Can you work these out from the model? Positions are in its coordinate system, mm. Face numbers are marked on the shaded views. A direction names the side the tool comes from. Round coordinates to 2 decimals unless told otherwise and drop trailing zeros. Order: outer loops, then holes, each group sorted by start corner. A loop starts at its lowest first (then second) coordinate and runs counter-clockwise, first axis right, second up. Notation, with made-up numbers: (-18.75, 69) - (35.25, 69) arc R15 cw to (35.25, 77) - close; hole circle Ø9 at (40, 73.25). An arc over 180 degrees is marked (long way). Write item = value, one per line.
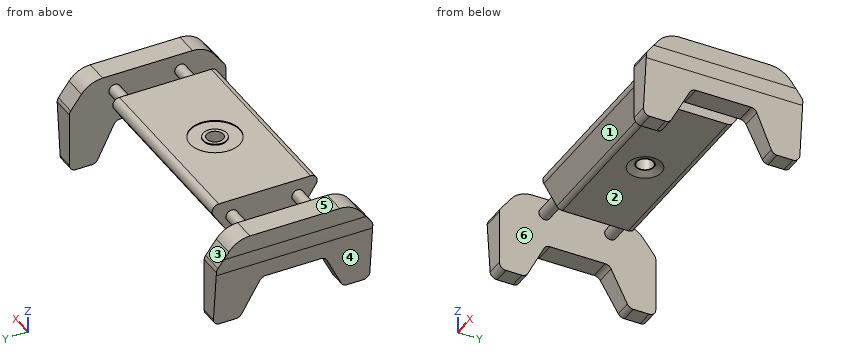
from build123d import *

# Parameters (mm, degrees)
BOSS_EXTRUDE1_DEPTH     = 56
SKETCH2_R               = 1.75
BOSS_EXTRUDE2_DEPTH     = 10
BOSS_EXTRUDE3_DEPTH     = 7
CUT_EXTRUDE1_DEPTH      = 13
CUT_EXTRUDE1_DEPTH_BACK = 44
FILLET1_R               = 45
CUT_EXTRUDE2_DEPTH      = 44
CUT_EXTRUDE2_DEPTH_BACK = 44
SKETCH5_R               = 2.5
SKETCH6_R               = 5
CUT_EXTRUDE3_DEPTH      = 1
CUT_EXTRUDE3_DRAFT      = -66
SKETCH7_R               = 7.5
SKETCH7_R_2             = 3.552716841
CUT_EXTRUDE4_DEPTH      = 0.3


with BuildPart() as part:
    # Sketch1 → Boss-Extrude1 (new body)
    with BuildSketch(Plane(origin=(0, 0, 0), x_dir=(0, 0, -1), z_dir=(1, 0, 0))):
        with BuildLine():
            Line((3.089976701, -2.008484856), (9.089976701, -5.908484856))
            ThreePointArc((9.089976701, -5.908484856), (9.757832956, -6.631420675), (10, -7.585372088))
            Line((10, -7.585372088), (10, -27.414627912))
            ThreePointArc((10, -27.414627912), (9.757832956, -28.368579325), (9.089976701, -29.091515144))
            Line((9.089976701, -29.091515144), (3.089976701, -32.991515144))
            ThreePointArc((3.089976701, -32.991515144), (1.046048587, -33.072460868), (0, -31.314627912))
            Line((0, -31.314627912), (0, -3.685372088))
            ThreePointArc((0, -3.685372088), (1.046048587, -1.927539132), (3.089976701, -2.008484856))
        make_face()
    extrude(amount=BOSS_EXTRUDE1_DEPTH)

    # Sketch2 → Boss-Extrude2 (add)
    with BuildSketch(Plane(origin=(56, 0, 0), x_dir=(0, 0, -1), z_dir=(1, 0, 0))):
        with Locations((5, -7.585372088)):
            Circle(SKETCH2_R)
        with Locations(Location((5, -27.414627912, 0), (0, 0, 180))):
            Circle(SKETCH2_R)
    extrude(amount=BOSS_EXTRUDE2_DEPTH)

    # Sketch3 → Boss-Extrude3 (add)
    with BuildSketch(Plane(origin=(66, 0, 0), x_dir=(0, 0, -1), z_dir=(1, 0, 0))):
        with BuildLine():
            Line((25.894427191, -32.489269358), (16.105572809, -27.594842167))
            ThreePointArc((16.105572809, -27.594842167), (15.298698383, -26.857450009), (15, -25.805987785))
            Line((15, -25.805987785), (15, -9.194012215))
            ThreePointArc((15, -9.194012215), (15.298698383, -8.142549991), (16.105572809, -7.405157833))
            Line((16.105572809, -7.405157833), (25.894427191, -2.510730642))
            ThreePointArc((25.894427191, -2.510730642), (26.701301617, -1.773338484), (27, -0.72187626))
            Line((27, -0.72187626), (27, 4.042055763))
            ThreePointArc((27, 4.042055763), (26.414213562, 5.456269325), (25, 6.042055763))
            Line((25, 6.042055763), (8.670397624, 6.042055763))
            ThreePointArc((8.670397624, 6.042055763), (8.034759221, 5.938358434), (7.465034823, 5.638019584))
            Line((7.465034823, 5.638019584), (3.178548798, 2.400621135))
            ThreePointArc((3.178548798, 2.400621135), (0.838589189, -0.417537137), (0, -3.98323415))
            Line((0, -3.98323415), (0, -31.01676585))
            ThreePointArc((0, -31.01676585), (0.838589189, -34.582462863), (3.178548798, -37.400621135))
            Line((3.178548798, -37.400621135), (7.465034823, -40.638019584))
            ThreePointArc((7.465034823, -40.638019584), (8.034759221, -40.938358434), (8.670397624, -41.042055763))
            Line((8.670397624, -41.042055763), (25, -41.042055763))
            ThreePointArc((25, -41.042055763), (26.414213562, -40.456269325), (27, -39.042055763))
            Line((27, -39.042055763), (27, -34.27812374))
            ThreePointArc((27, -34.27812374), (26.701301617, -33.226661516), (25.894427191, -32.489269358))
        make_face()
    extrude(amount=BOSS_EXTRUDE3_DEPTH)

    # Sketch4 → Cut-Extrude1 (cut, two sides: drawn at the far end of the back side and taken through both)
    with BuildSketch(Plane(origin=(0, 0, 0), x_dir=(1, 0, 0), z_dir=(0, 1, 0)).offset(-CUT_EXTRUDE1_DEPTH_BACK)):
        Polygon((73, 7.465034823), (71, 27), (73.488916827, 29.217701415), (75.731950279, 28.881788193), (75.634427086, 22.987052936), (74.610433553, 7.640140994), align=None)
    extrude(amount=CUT_EXTRUDE1_DEPTH + CUT_EXTRUDE1_DEPTH_BACK, mode=Mode.SUBTRACT)

    # Fillet1
    # the kernel refuses this fillet: 45 mm, written as the material it takes off along each edge
    with BuildSketch(Plane(origin=(73, -46.381911836, -7.465034823), x_dir=(0, 0, 1), z_dir=(0, 1, 0))) as fillet1_piece_1:
        with BuildLine():
            CenterArc((FILLET1_R * 0.0510568200202, -FILLET1_R), FILLET1_R, 90, 5.845604693)
            Line((-FILLET1_R * 0.0507913223976, -FILLET1_R * 0.00520004227682), (0, 0))
            Line((0, 0), (FILLET1_R * 0.0510568200202, 0))
        make_face()
    extrude(amount=57.763823673, mode=Mode.SUBTRACT)

    # Mirror1: part across plane


with BuildPart() as part_1:
    add(part.part)
    add(part.part.mirror(Plane(origin=(28, 0, 0), x_dir=(0, 0, 1), z_dir=(1, 0, 0))))

    # Sketch5 → Cut-Extrude2 (cut, two sides: drawn at the far end of the back side and taken through both)
    with BuildSketch(Plane.XY.offset(-CUT_EXTRUDE2_DEPTH_BACK)):
        with Locations(Location((28, -17.5, 0), (0, 0, 270))):
            Circle(SKETCH5_R)
    extrude(amount=CUT_EXTRUDE2_DEPTH + CUT_EXTRUDE2_DEPTH_BACK, mode=Mode.SUBTRACT)


with BuildPart() as cut_extrude3_tool:
    # Sketch6 → Cut-Extrude3 (with draft: the straight prism first)
    with BuildSketch(Plane(origin=(0, 0, -10), x_dir=(-1, 0, 0), z_dir=(0, 0, -1))):
        with Locations((-28, -17.5)):
            Circle(SKETCH6_R)
    extrude(amount=-CUT_EXTRUDE3_DEPTH)
    # Cut-Extrude3: the draft: its side faces are tilted about the plane it starts from
    cut_extrude3_sides = [cut_extrude3_tool.faces().sort_by_distance(p)[0] for p in [
        (33, -17.5, -9.5),
    ]]
    draft(cut_extrude3_sides, Plane(origin=(0, 0, -10), x_dir=(-1, 0, 0), z_dir=(0, 0, -1)), CUT_EXTRUDE3_DRAFT)


with BuildPart() as part_2:
    add(part_1.part)

    # Cut-Extrude3: cut by cut_extrude3_tool
    add(cut_extrude3_tool.part, mode=Mode.SUBTRACT)

    # Sketch7 → Cut-Extrude4 (cut)
    with BuildSketch(Plane.XY):
        with Locations((28, -17.5)):
            Circle(SKETCH7_R)
        with Locations((28, -17.5)):
            Circle(SKETCH7_R_2, mode=Mode.SUBTRACT)
    extrude(amount=-CUT_EXTRUDE4_DEPTH, mode=Mode.SUBTRACT)


solid = part_2.part
(1) If I drill on line 1 (X direction, y = -17.5, z = -5); line 2 (X direction, y = -11, z = -7); line 3 (X direction, y = 3, z = -5.25), over which ranges is the centre line in solid material (lowest first)? Write a range as from..to.
Computed:
line_1 = -17..-10, 0..25.5, 30.5..56, 66..73
line_2 = -16.96..-10, 0..56, 66..72.96
line_3 = -17..-10, 66..73
(2) If we section it at D-D (x = 39): Write out the boundary of the cut face in (y, z), plus the area to 3 significant figures.
Computed:
outline = (-32.99, -3.09) - (-29.09, -9.09) arc R2 ccw to (-27.41, -10) - (-7.59, -10) arc R2 ccw to (-5.91, -9.09) - (-2.01, -3.09) arc R2 ccw to (-3.69, 0) - (-31.31, 0) arc R2 ccw to start
area = 278 mm^2
(3) If we section it at C-C (z = -19.75): Write out the boundary of the cut face in (x, y).
Computed:
outline = (-15.74, -41.04) - (-10, -41.04) - (-10, -29.42) - (-15.74, -29.42) - close; (-15.74, -5.58) - (-10, -5.58) - (-10, 6.04) - (-15.74, 6.04) - close; (66, -41.04) - (71.74, -41.04) - (71.74, -29.42) - (66, -29.42) - close; (66, -5.58) - (71.74, -5.58) - (71.74, 6.04) - (66, 6.04) - close
(4) If we section it at A-A (y = -17.5): State how many separate pieces and enclosed holes the cut face has, plus the area to 3 significant figures.
Computed:
separate_pieces = 4
enclosed_holes = 0
area = 709 mm^2
(5) Thinking about a two-plate mould opening in X: for the marked faces 4, 5 and 6, which applies, +X half, -X half, draft (parallel to the pull), parting line (faces both ways), or undercut?
Computed:
face_4 = -X half
face_5 = draft
face_6 = undercut
(6) If we section it at B-B (x = 28): Write out the boundary of the cut face in (y, z).
Computed:
outline = (-32.99, -3.09) - (-29.09, -9.09) arc R2 ccw to (-27.41, -10) - (-22.5, -10) - (-20.25, -9) - (-20, -9) - (-20, 0) - (-21.05, 0) - (-21.05, -0.3) - (-25, -0.3) - (-25, 0) - (-31.31, 0) arc R2 ccw to start; (-15, -9) - (-14.75, -9) - (-12.5, -10) - (-7.59, -10) arc R2 ccw to (-5.91, -9.09) - (-2.01, -3.09) arc R2 ccw to (-3.69, 0) - (-10, 0) - (-10, -0.3) - (-13.95, -0.3) - (-13.95, 0) - (-15, 0) - close
(7) On a 3-axis mill with a long thin cutter (end or side, diameter ignored), from which of +Z, -Z, +X, -X, +Y, -Y can I reach the whole of each face in a straight line? I mean the marked faces 1, 2 and 3. Say none if no direction works.
Computed:
face_1 = -Z, -Y
face_2 = -Z, +Y, -Y
face_3 = +Z, +X, -X, +Y
(8) Will these pins go through, and if not, where does the flat tip stop? P1, Ø7, axis at x = 70, y = -16, coming from the -Z side; P2, Ø10, axis at x = 56, z = -15.5, coming from the +Y side; P3, Ø16, axis at x = 40.5, y = -17.5, coming from the -Z side; P4, Ø8, axis at x = 28, y = -17.5, coming from the -Z side.
Computed:
P1 = -15
P2 = through
P3 = -10
P4 = -9.55
